Part print with two shaded views. Sizes in mm from the minimum x, y, z corner. A direction names the side the tool comes from. Give positions to 0.01 mm unless a question says otherwise; leave off trailing zeros. Order: outer loops, then holes, each group sorted by start corner. A loop starts at its lowest first (then second) coordinate and runs counter-clockwise, first axis right, second up. Notation, with made-up numbers: M 39.5,-28 L 53.5,-28 A10 ccw 53.5,-9 Z; hole C -38.5,0.5 d11. An arc over 180 degrees is marked long. Answer as CSV lines item,"result".
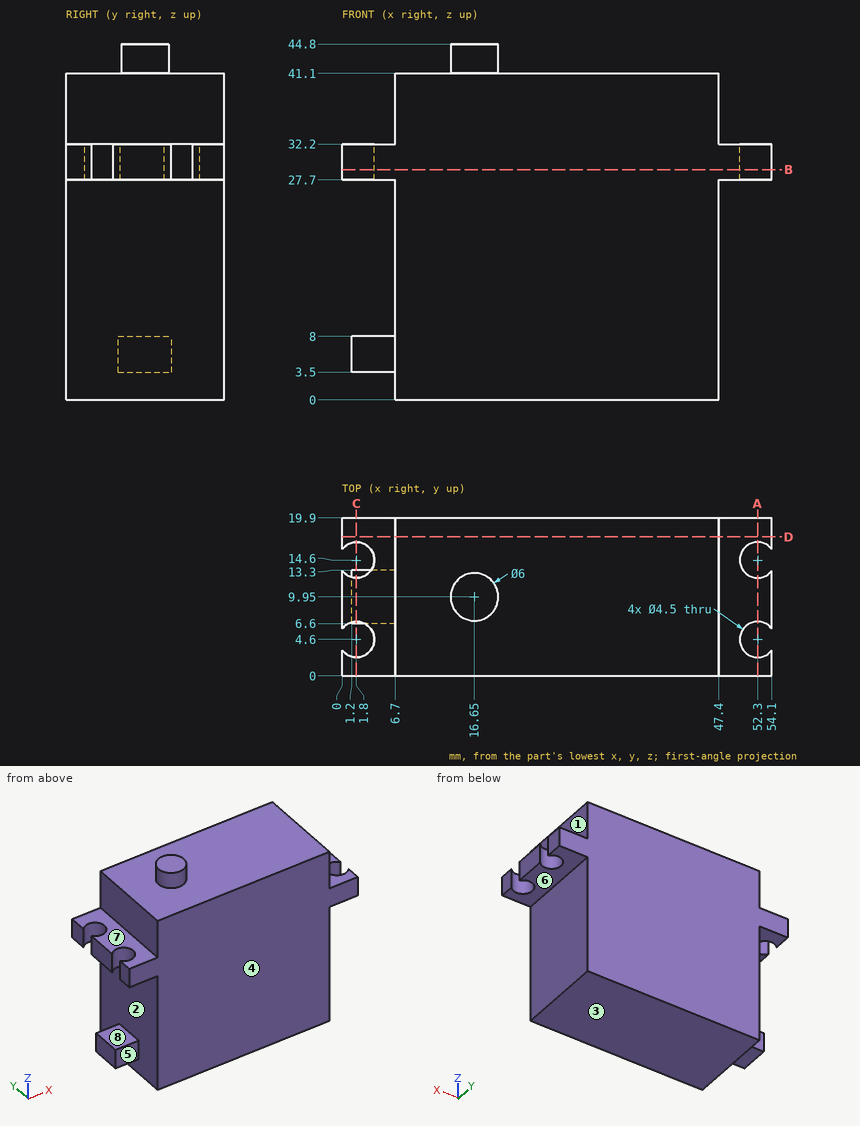
Item 1: Probe line 1 along Y through (x, z) = (1.8, 29.45); line 2 along Y through (x, z) = (52, 29); line 3 along Z through (x, y) = (5.5, 7.25). List the from-to ranges inside material, lowest first. Write a range as from..to.
Geometry says:
line 1,"y = 0..2.35, 6.85..12.35, 16.85..19.9"
line 2,"y = 0..2.37, 6.83..12.37, 16.83..19.9"
line 3,"z = 3.5..8, 27.7..32.2"
Item 2: Band-saw the part on C-C (x = 1.8). Give the cut face in (y, z).
Geometry says:
outline,"M 0,27.7 L 2.35,27.7 L 2.35,32.2 L 0,32.2 Z; M 6.6,3.5 L 13.3,3.5 L 13.3,8 L 6.6,8 Z; M 6.85,27.7 L 12.35,27.7 L 12.35,32.2 L 6.85,32.2 Z; M 16.85,27.7 L 19.9,27.7 L 19.9,32.2 L 16.85,32.2 Z"
Item 3: Pull direction Z, two halves, no side cores. Call the marked faces 1, 2 and 3: released by +Z, released by -Z, zero draft, split by the parting line, or undercut.
Geometry says:
face 1,"zero draft"
face 2,"undercut"
face 3,"released by -Z"
Item 4: Band-saw the part on B-B (z = 29). Give the cut face in (x, y).
Geometry says:
outline,"M 0,0 L 54.1,0 L 54.1,3.25 A2.25 cw long 54.1,5.95 L 54.1,13.25 A2.25 cw long 54.1,15.95 L 54.1,19.9 L 0,19.9 L 0,15.95 A2.25 cw long 0,13.25 L 0,5.95 A2.25 cw long 0,3.25 Z"
Item 5: 3-axis set-ups, long thin cutter, end or side, ignore diameter. For the marked faces 4, 5, 6, 7 and 8: which of +Z, -Z, +X, -X, +Y, -Y reach the whole face in a straight line?
Geometry says:
face 4,"+Z, -Z, +X, -X, -Y"
face 5,"-Z, -X, -Y"
face 6,"-Z, +X, +Y, -Y"
face 7,"+Z, -X, +Y, -Y"
face 8,"-X, +Y, -Y"
Item 6: Band-saw the part on D-D (y = 17.5). Give the cut face in (x, z), and give its area (3 significant figures).
Geometry says:
outline,"M 0,27.7 L 6.7,27.7 L 6.7,0 L 47.4,0 L 47.4,27.7 L 54.1,27.7 L 54.1,32.2 L 47.4,32.2 L 47.4,41.1 L 6.7,41.1 L 6.7,32.2 L 0,32.2 Z"
area,"1,730 mm2"
Item 7: Band-saw the part on A-A (x = 52.3). Give the cut face in (y, z).
Geometry says:
outline,"M 0,27.7 L 2.35,27.7 L 2.35,32.2 L 0,32.2 Z; M 6.85,27.7 L 12.35,27.7 L 12.35,32.2 L 6.85,32.2 Z; M 16.85,27.7 L 19.9,27.7 L 19.9,32.2 L 16.85,32.2 Z"
Item 8: Drop flat-ended pins along their axis: pin 1 (5 mm diameter, centred on x = 5, z = 6, fed in from -Y); pin 2 (2.5 mm diameter, centred on x = 1.8, y = 4.6, fed in from -Z); pin 3 (1.7 mm diameter, centred on x = 3, y = 9.5, fed in from +Z); pin 4 (1.7 mm diameter, centred on x = 5, y = 10, fed in from -Z). Give the stop position or say it passes through.
Geometry says:
pin 1,"stops at y = 0"
pin 2,"passes through"
pin 3,"stops at z = 32.2"
pin 4,"stops at z = 3.5"
